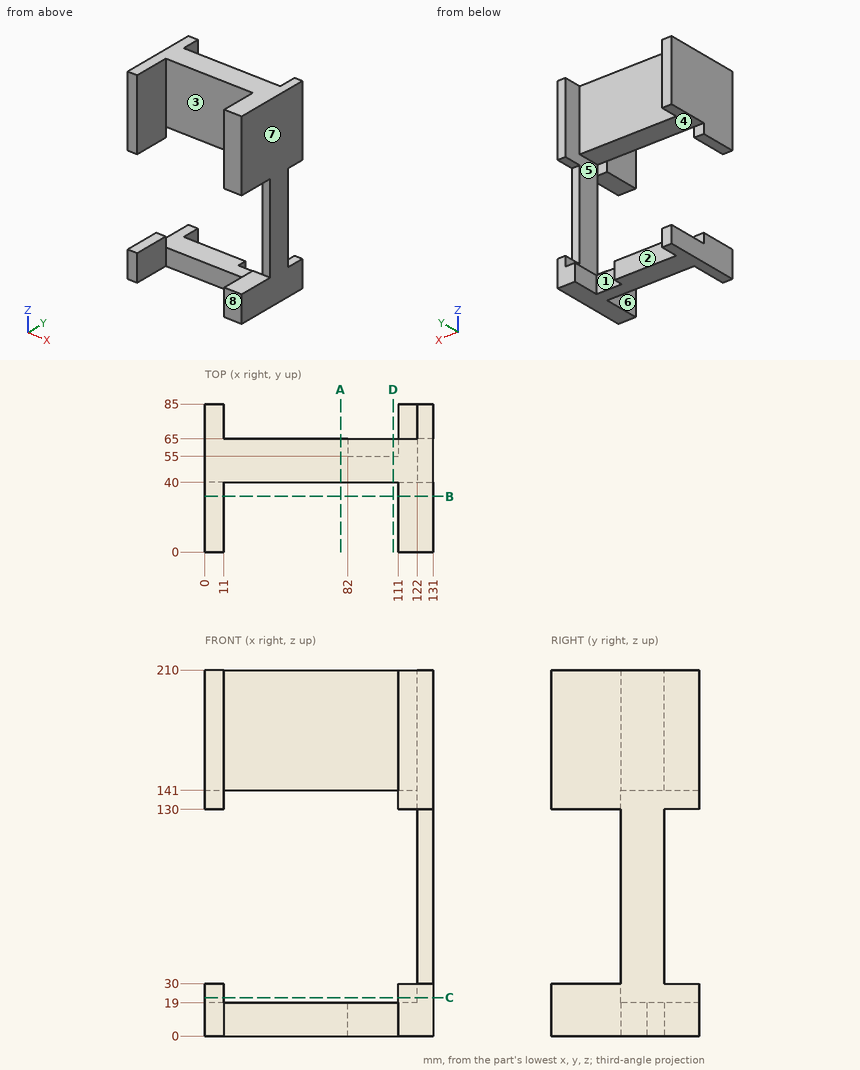
Drawing for the job (mm, zero at the part's lowest x, y, z). A direction names the side the tool comes from. Round coordinates to 2 decimals unless told otherwise and drop trailing zeros. Write each loop counter-clockwise with the first axis right and the second up, starting at its lowest first coordinate (ties: lowest second). Pieces come first, ordered by that corner, then holes. Notation, with made-up numbers: (0, 30.25) - (7, 30.25) arc R25 ccw to (7, 61.25) - close; hole circle Ø5 at (39, -14.75). An arc over 180 degrees is marked (long way). Return JSON: item names as keys, results as strings. Group by question number.
Item 1: Probe probe 1 along X at (y, z) = (70.5, 176); probe 2 along X at (y, z) = (23.5, 199); probe 3 along Z at (x, y) = (39, 51). List the from-to ranges inside material, lowest first.
Item 2: Band-saw the part on D-D on x = 108. List the corners of the cut face in (y, z).
Item 3: Flat gauge pins, fed straight in: pin 1 Ø4 at (y, z) = (61, 94.5) entering from -X; pin 2 Ø7 at (x, z) = (126.5, 81.5) entering from +Y; pin 3 Ø12 at (x, z) = (7, 26.5) entering from +Y. Where does each tip first touch, or does it go through?
Item 4: Band-saw the part on C-C on z = 22. List the corners of the cut face in (x, y).
Item 5: Mould opens along X. For the marked faces 5, 6, 7 and 8 say: +X half, -X half, draft (parallel to the pull), parting line (faces both ways), or undercut.
Item 6: 3-axis set-ups, long thin cutter, end or side, ignore diameter. For the marked faces 1, 2, 3 and 4: which of +Z, -Z, +X, -X, +Y, -Y reach the whole face in a straight line?
Item 7: Band-saw the part on A-A on x = 78. List the corners of the cut face in (y, z), plus the area to 3 significant figures.
Item 8: Band-saw the part on B-B on y = 32. List the corners of the cut face in (x, z).
Resolved:
{
 "1": {"probe 1": "x = 0 to 11, 122 to 131", "probe 2": "x = 0 to 11, 111 to 131", "probe 3": "z = 0 to 19, 141 to 210"},
 "2": {"outline": "(40, 0) - (55, 0) - (55, 19) - (40, 19) - close; (40, 141) - (65, 141) - (65, 210) - (40, 210) - close"},
 "3": {"pin 1": "stops at x = 122", "pin 2": "stops at y = 65", "pin 3": "stops at y = 40"},
 "4": {"outline": "(0, 0) - (11, 0) - (11, 40) - (0, 40) - close; (111, 0) - (131, 0) - (131, 85) - (122, 85) - (122, 40) - (111, 40) - close"},
 "5": {"face 5": "undercut", "face 6": "undercut", "face 7": "+X half", "face 8": "draft"},
 "6": {"face 1": "-Z, +Y", "face 2": "+Z, -Z, +Y", "face 3": "+Z, -Z, -Y", "face 4": "-X, +Y"},
 "7": {"outline": "(40, 0) - (65, 0) - (65, 19) - (40, 19) - close; (40, 141) - (65, 141) - (65, 210) - (40, 210) - close", "area": "2,200 mm²"},
 "8": {"outline": "(0, 0) - (11, 0) - (11, 30) - (0, 30) - close; (0, 130) - (11, 130) - (11, 210) - (0, 210) - close; (111, 0) - (131, 0) - (131, 30) - (111, 30) - close; (111, 130) - (131, 130) - (131, 210) - (111, 210) - close"}
}
